Read the model definition and answer for the solid it produces. Units are mm, in the model's axes. Face numbers are marked on the shaded views. A direction names the side the tool comes from. Coordinates: 2 decimals unless noted, no trailing zeros. Loops run counter-clockwise (first coordinate to the right, second up) from the corner with the lowest first, then second, coordinate; pieces in that order, holes last. Notation, with made-up numbers: M 27,-16.75 L 42,-16.75 A8 ccw 42,-10.75 Z; hole C 89,74 d1. An arc over 180 degrees is marked long. Put each result on its own line as item: value.
from build123d import *

# Parameters (mm, degrees)
SKETCH1_R           = 22
BOSS_EXTRUDE1_DEPTH = 14
SKETCH2_R           = 24
BOSS_EXTRUDE2_DEPTH = 9
SKETCH3_R           = 32
BOSS_EXTRUDE3_DEPTH = 9
SKETCH5_R           = 4
BOSS_EXTRUDE4_DEPTH = 30
CUT_EXTRUDE2_REACH  = 66
SKETCH4_R           = 16
SKETCH6_R           = 3
CUT_EXTRUDE3_DEPTH  = 63


with BuildPart() as part:
    # Sketch1 → Boss-Extrude1 (new body, symmetric)
    with BuildSketch(Plane.XY):
        Circle(SKETCH1_R)
    extrude(amount=BOSS_EXTRUDE1_DEPTH, both=True)

    # Sketch2 → Boss-Extrude2 (add)
    with BuildSketch(Plane.XY.offset(14)):
        Circle(SKETCH2_R)
    boss_extrude2 = extrude(amount=BOSS_EXTRUDE2_DEPTH)

    # Mirror1: Boss-Extrude2 across plane
    add(boss_extrude2.mirror(Plane.XY))

    # Sketch3 → Boss-Extrude3 (add)
    with BuildSketch(Plane.XY.offset(23)):
        Circle(SKETCH3_R)
    boss_extrude3 = extrude(amount=BOSS_EXTRUDE3_DEPTH)

    # Mirror2: Boss-Extrude3 across plane
    add(boss_extrude3.mirror(Plane.XY))

    # Sketch5 → Boss-Extrude4 (add)
    with BuildSketch(Plane(origin=(0, 0, 0), x_dir=(1, 0, 0), z_dir=(0, 1, 0))):
        Circle(SKETCH5_R)
    extrude(amount=-BOSS_EXTRUDE4_DEPTH)

    # Sketch4 → Cut-Extrude2 (cut, up to next)
    with BuildSketch(Plane.XY.offset(32), mode=Mode.PRIVATE) as cut_extrude2_sk1:
        Circle(SKETCH4_R)
    cut_extrude2_tool1 = extrude(cut_extrude2_sk1.sketch, amount=-CUT_EXTRUDE2_REACH, mode=Mode.PRIVATE) & part.part
    add(cut_extrude2_tool1.solids().sort_by_distance((0, 0, 32))[0], mode=Mode.SUBTRACT)

    # Sketch6 → Cut-Extrude3 (cut, through all)
    with BuildSketch(Plane.XZ.offset(30)):
        Circle(SKETCH6_R)
    extrude(amount=-CUT_EXTRUDE3_DEPTH, mode=Mode.SUBTRACT)


solid = part.part
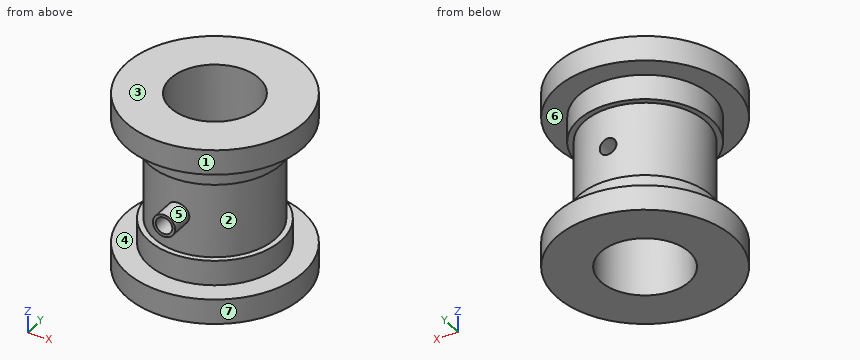
1) Find section D-D, the plane y = -23. Write down the section's boundary in (x, z).
Answer list:
outline: M -22.25,-32 L 22.25,-32 L 22.25,-23 L 6.86,-23 L 6.86,-14 L -6.86,-14 L -6.86,-23 L -22.25,-23 Z; M -22.25,23 L -6.86,23 L -6.86,14 L 6.86,14 L 6.86,23 L 22.25,23 L 22.25,32 L -22.25,32 Z; C 0,0 d8; hole C 0,0 d6
2) Find section C-C, the plane z = 1. Write down the section's boundary in (x, y), plus the area to 3 significant figures.
Answer list:
outline: M -3.87,-30 L -2.83,-30 L -2.83,-15.75 A16 cw -2.83,15.75 L -2.83,21.82 A22 ccw -3.87,-21.66 Z; M 2.83,-30 L 3.87,-30 L 3.87,-21.66 A22 ccw 2.83,21.82 L 2.83,15.75 A16 cw 2.83,-15.75 Z
area: 665 mm^2
3) Which of the six approach directions +Z, -Z, +X, -X, +Y, -Y give full straight-line access (tool end or side, diameter ignored) to the marked faces 5, 6 and 7?
Answer list:
face 5: -Y
face 6: none
face 7: +Z, -Z
4) Find section A-A, the plane y = 0. Write down the section's boundary in (x, z), plus the area to 3 significant figures.
Answer list:
outline: M -32,-32 L -16,-32 L -16,32 L -32,32 L -32,23 L -24,23 L -24,14 L -22,14 L -22,-14 L -24,-14 L -24,-23 L -32,-23 Z; M 16,-32 L 32,-32 L 32,-23 L 24,-23 L 24,-14 L 22,-14 L 22,14 L 24,14 L 24,23 L 32,23 L 32,32 L 16,32 Z
area: 1,200 mm^2
5) Determine the mould class of the marked faces 1, 2, 3 and 4 for opening direction Z: released by +Z, released by -Z, zero draft, split by the parting line, or undercut.
Answer list:
face 1: zero draft
face 2: undercut
face 3: released by +Z
face 4: undercut
6) Straight lines are drawn through the part: line 1 (Z direction, x = 0, y = -25.5); line 2 (Z direction, x = 0, y = -18.75); line 3 (Z direction, x = 27.5, y = 0.5). For each, find the intervals that lie inside material, in ascending order. Write a range as [from, to].
Answer list:
line 1: z = [-32, -23], [-4, -3], [3, 4], [23, 32]
line 2: z = [-32, -3], [3, 32]
line 3: z = [-32, -23], [23, 32]
7) Find section B-B, the plane x = -14. Write down the section's boundary in (y, z), plus the area to 3 significant figures.
Answer list:
outline: M -28.77,-32 L -7.75,-32 L -7.75,32 L -28.77,32 L -28.77,23 L -19.49,23 L -19.49,14 L -16.97,14 L -16.97,-14 L -19.49,-14 L -19.49,-23 L -28.77,-23 Z; M 7.75,-32 L 28.77,-32 L 28.77,-23 L 19.49,-23 L 19.49,-14 L 16.97,-14 L 16.97,14 L 19.49,14 L 19.49,23 L 28.77,23 L 28.77,32 L 7.75,32 Z
area: 1,700 mm^2
8) Given pin 1 Ø6.5 at (x, z) = (2, 0) entering from -Y; pin 2 Ø6 at (x, z) = (22.5, 13.5) entering from +Y; pin 3 Ø14.5 at (x, y) = (-1.5, -0.5) entering from -Z; pin 4 Ø8 at (x, z) = (0, 0) entering from +Y, each flat-ended and moving along its own axis, determine where each tip first touches the part or whether it passes through.
Answer list:
pin 1: stops at y = -30
pin 2: stops at y = 13.93
pin 3: passes through
pin 4: stops at y = 22
